Source: CAD feature listing. Evaluate the final solid. Frame: model axes, mm. A direction names the side the tool comes from. Give positions to 0.01 mm unless a question says otherwise; leave off trailing zeros. Loops run counter-clockwise (first coordinate to the right, second up) from the corner with the lowest first, then second, coordinate; pieces in that order, holes last. Notation, with made-up numbers: (81.5, 73) -> (139.5, 73) arc R5 ccw to (139.5, 77) -> close; hole circle Ø4 at (-16, 23.25). An arc over 180 degrees is marked (long way). Return JSON: item names as keys, results as strings. Group by question number.
(1) Draft query along Y for faces 1 (the face through (468, 725, 7)), 2 (the face through (245.66, 750, 14)), 3 (the face through (468, 727, 6)). Return one class per face: released by +Y, released by -Y, zero draft, split by the parting line, or undercut.
(2) Cut plane B-B on y = 749.5. Return loops of the section in (x, z), then the cut area to 3 significant figures.
(3) Access query for faces 4 (the face through (269.58, 744.62, 14.01)), 5 (the face through (468, 745, 13)). Directions: +Z, -Z, +X, -X, +Y, -Y. A direction counts if a zero-diameter tool reaches every point of the face in a straight line with its end or side. Return the directions, or none.
(4) Cut plane A-A on z = 7.5. Return loops of the section in (x, y).
(5) Pin query (flat end, axial travel): pin 1 (13 mm diameter, centred on x = 514, y = 746.5, fed in from -Z); pin 2 (8 mm diameter, centred on x = 470.66, y = 749.5, fed in from +Z). Return the tip coordinate at first contact, or that it passes through.
(6) Ray query, line 1 (X direction, y = 749.5, z = 13.5); line 2 (Y direction, x = 268, z = 9.5); line 3 (X direction, y = 747.5, z = 14.25). Return the intervals inside material, ascending. Write a range as from..to.
(7) Cut plane D-D on y = 732.5. Return loops of the section in (x, z).
Autodesk Inventor part; units mm, degrees
ref_plane "Work Plane1" through (0, 0, 0) normal (0, 0, 1) x (1, 0, 0)
ref_plane "YZ Plane" through (0, 0, 0) normal (1, 0, 0) x (0, 1, 0)
ref_plane "XZ Plane" through (0, 0, 0) normal (0, 1, 0) x (-1, 0, 0)
ref_plane "Work Plane1" through (0, 0, 0) normal (0, 0, 1) x (1, 0, 0)
sketch "Sketch1" plane through (0, 0, 0) normal (0, 0, 1) x (1, 0, 0)
  line L0 (245.6597, 725) -> (695.6597, 725)
  line L1 (695.6597, 725) -> (695.6597, 775)
  line L2 (695.6597, 775) -> (245.6597, 775)
  line L3 (245.6597, 775) -> (245.6597, 725)
  line L4 (164.0316, 10) -> (164.0316, 1490)
  line L5 (777.2877, 10) -> (164.0316, 10)
  line L6 (470.6597, 10) -> (470.6597, 1506) construction
  line L7 (164.0316, 750) -> (680, 750) construction
  point P0 (0, 0)
  point P1 (470.6597, 725)
  point P2 (245.6597, 750)
  dimension "d0" = 450
  dimension "d1" = 50
extrude "Extrusion1" add sketch "Sketch1" along normal blind 15
sketch "Sketch2" plane through (245.6597, 725, 0) normal (-1, 0, 0) x (0, 0, 1)
  line L0 (15, 0) -> (0, 0)
  line L1 (0, 0) -> (0, 50)
  line L2 (0, 50) -> (15, 50)
  line L3 (15, 50) -> (15, 0)
  line L4 (12, 48) -> (0, 48)
  line L5 (0, 2) -> (12, 2)
  line L6 (13, 3) -> (13, 47)
  arc A0 (13, 47) -> (12, 48) centre (12, 47) ccw
  arc A1 (12, 2) -> (13, 3) centre (12, 3) ccw
  point P0 (0, -725)
  dimension "d5" = 2
extrude "Extrusion2" cut sketch "Sketch2" against normal through all contours L1 L4 A0 L6 A1 L5
fillet "Fillet1" radius 2 4 edges at (470.6597, 775, 15) (470.6597, 775, 0) (470.6597, 725, 0) (470.6597, 725, 15)
sketch "Sketch3" plane through (0, 0, 15) normal (0, 0, 1) x (1, 0, 0)
  line L0 (245.6597, 727) -> (695.6597, 727) construction
  line L1 (695.6597, 773) -> (695.6597, 727) construction
  line L2 (695.6597, 773) -> (245.6597, 773) construction
  line L3 (245.6597, 727) -> (245.6597, 773) construction
  line L4 (245.6597, 772) -> (695.6597, 772)
  line L5 (470.6597, 772) -> (470.6597, 727) construction
  circle A0 centre (470.6597, 749.5) radius 5
  point P0 (0, 0)
  dimension "d10" = 10
extrude "Extrusion3" cut sketch "Sketch3" against normal up to next
pattern_linear "Rectangular Pattern1" count 5 spacing 100 along (1, 0, 0) of "Extrusion3" first direction both ways yes
properties part number "support1" material "Stainless Steel"
Answers:
{
 "1": {"face 1": "released by -Y", "face 2": "zero draft", "face 3": "undercut"},
 "2": {"outline": "(245.66, 13) -> (265.66, 13) -> (265.66, 15) -> (245.66, 15) -> close; (275.66, 13) -> (365.66, 13) -> (365.66, 15) -> (275.66, 15) -> close; (375.66, 13) -> (465.66, 13) -> (465.66, 15) -> (375.66, 15) -> close; (475.66, 13) -> (565.66, 13) -> (565.66, 15) -> (475.66, 15) -> close; (575.66, 13) -> (665.66, 13) -> (665.66, 15) -> (575.66, 15) -> close; (675.66, 13) -> (695.66, 13) -> (695.66, 15) -> (675.66, 15) -> close", "area": "800 mm²"},
 "3": {"face 4": "+Z, -Z", "face 5": "-Z, +X, -X"},
 "4": {"outline": "(245.66, 725) -> (695.66, 725) -> (695.66, 727) -> (245.66, 727) -> close; (245.66, 773) -> (695.66, 773) -> (695.66, 775) -> (245.66, 775) -> close"},
 "5": {"pin 1": "z = 13", "pin 2": "through"},
 "6": {"line 1": "245.66..265.66, 275.66..365.66, 375.66..465.66, 475.66..565.66, 575.66..665.66, 675.66..695.66", "line 2": "725..727, 773..775", "line 3": "245.66..266.08, 275.24..366.08, 375.24..466.08, 475.24..566.08, 575.24..666.08, 675.24..695.66"},
 "7": {"outline": "(245.66, 13) -> (695.66, 13) -> (695.66, 15) -> (245.66, 15) -> close"}
}
